Geometry: final body of the model. Coordinates: model frame, mm. Give positions to 0.01 mm unless a question says otherwise; leave off trailing zeros. Write each loop counter-clockwise with the first axis right and the second up, starting at its lowest first coordinate (ties: lowest second). Pieces come first, ordered by that corner, then holes.
Q1. Pin query (flat end, axial travel): pin 1 (1 mm diameter, centred on y = -37.5, z = 1, fed in from -X); pin 2 (0.6 mm diameter, centred on y = -33.5, z = 0.5, fed in from +X); pin 3 (0.6 mm diameter, centred on x = 16, z = 1.5, fed in from -Y). Return the tip coordinate at first contact, or that it passes through.
Q2. Line query: L1, parallel to Y at x = -22, z = 1.4; L2, parallel to X at y = -3.5, z = 0.5; L3, parallel to Y at x = 15, z = 0.5. Output: solid intervals per line, ascending.
Q3. Cut plane A-A on x = -16.5. Return the cut outline in (y, z).
Q4. Cut plane B-B on x = -22. Return the cut outline in (y, z).
Q5. Cut plane C-C on y = 2. Return the cut outline in (x, z).
Q6. Cut plane D-D on z = 1.35. Count the separate pieces of the cut face and the enclosed holes in it, plus the area to 3 significant figures.
```python
from build123d import *

# Parameters (mm, degrees)
F0_R     = 0.6
F0_R_2   = 0.85
F1_DEPTH = 2
F2_R     = 1


# Not quite as in the source:
# - a feature names something its author has since deleted; it is built from what else it names


with BuildPart() as f1:
    # F0 (on Top) → F1 (new body)
    with BuildSketch(Plane.XY):
        with BuildLine():
            ThreePointArc((-5.75, -27.5638593384), (-6.75, -27.25), (-7.75, -27.5638593384))
            Line((-7.75, -27.5638593384), (-7.75, -30.4361406616))
            ThreePointArc((-7.75, -30.4361406616), (-6.75, -30.75), (-5.75, -30.4361406616))
            Line((-5.75, -30.4361406616), (-5.75, -27.5638593384))
        make_face()
        with Locations((-6.75, -29)):
            Circle(F0_R, mode=Mode.SUBTRACT)
        with BuildLine():
            Line((-7.75, -30.4361406616), (-7.75, -27.5638593384))
            ThreePointArc((-7.75, -27.5638593384), (-8.5, -29), (-7.75, -30.4361406616))
        make_face()
        with BuildLine():
            ThreePointArc((-5.75, -30.4361406616), (-6.75, -30.75), (-7.75, -30.4361406616))
            Line((-7.75, -30.4361406616), (-7.75, -39.5638593384))
            ThreePointArc((-7.75, -39.5638593384), (-6.75, -39.25), (-5.75, -39.5638593384))
            Line((-5.75, -39.5638593384), (-5.75, -30.4361406616))
        make_face()
        with BuildLine():
            Line((-7.75, -42.4361406616), (-7.75, -39.5638593384))
            ThreePointArc((-7.75, -39.5638593384), (-8.5, -41), (-7.75, -42.4361406616))
        make_face()
        with BuildLine():
            ThreePointArc((-5.75, -39.5638593384), (-6.75, -39.25), (-7.75, -39.5638593384))
            Line((-7.75, -39.5638593384), (-7.75, -42.4361406616))
            ThreePointArc((-7.75, -42.4361406616), (-6.75, -42.75), (-5.75, -42.4361406616))
            Line((-5.75, -42.4361406616), (-5.75, -39.5638593384))
        make_face()
        with Locations((-6.75, -41)):
            Circle(F0_R, mode=Mode.SUBTRACT)
        with BuildLine():
            ThreePointArc((-5.75, -42.4361406616), (-6.75, -42.75), (-7.75, -42.4361406616))
            Line((-7.75, -42.4361406616), (-7.75, -46.5))
            Line((-7.75, -46.5), (7.75, -46.5))
            Line((7.75, -46.5), (7.75, -42.4361406616))
            ThreePointArc((7.75, -42.4361406616), (6.75, -42.75), (5.75, -42.4361406616))
            Line((5.75, -42.4361406616), (5.75, -45))
            Line((5.75, -45), (-5.75, -45))
            Line((-5.75, -45), (-5.75, -42.4361406616))
        make_face()
        with BuildLine():
            Line((7.75, -30.4361406616), (7.75, -27.5638593384))
            ThreePointArc((7.75, -27.5638593384), (6.75, -27.25), (5.75, -27.5638593384))
            Line((5.75, -27.5638593384), (5.75, -30.4361406616))
            ThreePointArc((5.75, -30.4361406616), (6.75, -30.75), (7.75, -30.4361406616))
        make_face()
        with Locations((6.75, -29)):
            Circle(F0_R, mode=Mode.SUBTRACT)
        with BuildLine():
            ThreePointArc((8.5, -29), (8.3012092057, -28.1899074127), (7.75, -27.5638593384))
            Line((7.75, -27.5638593384), (7.75, -30.4361406616))
            ThreePointArc((7.75, -30.4361406616), (8.3012092057, -29.8100925873), (8.5, -29))
        make_face()
        with BuildLine():
            Line((7.75, -39.5638593384), (7.75, -30.4361406616))
            ThreePointArc((7.75, -30.4361406616), (6.75, -30.75), (5.75, -30.4361406616))
            Line((5.75, -30.4361406616), (5.75, -39.5638593384))
            ThreePointArc((5.75, -39.5638593384), (6.75, -39.25), (7.75, -39.5638593384))
        make_face()
        with BuildLine():
            Line((7.75, -42.4361406616), (7.75, -39.5638593384))
            ThreePointArc((7.75, -39.5638593384), (6.75, -39.25), (5.75, -39.5638593384))
            Line((5.75, -39.5638593384), (5.75, -42.4361406616))
            ThreePointArc((5.75, -42.4361406616), (6.75, -42.75), (7.75, -42.4361406616))
        make_face()
        with Locations((6.75, -41)):
            Circle(F0_R, mode=Mode.SUBTRACT)
        with BuildLine():
            ThreePointArc((8.5, -41), (8.3012092057, -40.1899074127), (7.75, -39.5638593384))
            Line((7.75, -39.5638593384), (7.75, -42.4361406616))
            ThreePointArc((7.75, -42.4361406616), (8.3012092057, -41.8100925873), (8.5, -41))
        make_face()
        with BuildLine():
            ThreePointArc((-20, -8), (-20.0681483474, -8.5176380902), (-20.2679491924, -9))
            Line((-20.2679491924, -9), (-7.75, -9))
            Line((-7.75, -9), (-5.75, -9))
            Line((-5.75, -9), (5.75, -9))
            Line((5.75, -9), (7.75, -9))
            Line((7.75, -9), (20.2679491924, -9))
            ThreePointArc((20.2679491924, -9), (20, -8), (20.2679491924, -7))
            Line((20.2679491924, -7), (-20.2679491924, -7))
            ThreePointArc((-20.2679491924, -7), (-20.0681483474, -7.4823619098), (-20, -8))
        make_face()
        with BuildLine():
            ThreePointArc((24, -8), (23.7320508076, -7), (23, -6.2679491924))
            Line((23, -6.2679491924), (23, -9))
            Line((23, -9), (20.2679491924, -9))
            ThreePointArc((20.2679491924, -9), (22.5176380902, -9.9318516526), (24, -8))
        make_face()
        with BuildLine():
            ThreePointArc((23, -6.2679491924), (22, -6), (21, -6.2679491924))
            Line((21, -6.2679491924), (21, -7))
            Line((21, -7), (20.2679491924, -7))
            ThreePointArc((20.2679491924, -7), (20, -8), (20.2679491924, -9))
            Line((20.2679491924, -9), (23, -9))
            Line((23, -9), (23, -6.2679491924))
        make_face()
        with Locations((22, -8)):
            Circle(F0_R_2, mode=Mode.SUBTRACT)
        with BuildLine():
            ThreePointArc((23, 6.2679491924), (22, 6), (21, 6.2679491924))
            Line((21, 6.2679491924), (21, -6.2679491924))
            ThreePointArc((21, -6.2679491924), (22, -6), (23, -6.2679491924))
            Line((23, -6.2679491924), (23, 6.2679491924))
        make_face()
        with BuildLine():
            Line((21, -7), (21, -6.2679491924))
            ThreePointArc((21, -6.2679491924), (20.5857864376, -6.5857864376), (20.2679491924, -7))
            Line((20.2679491924, -7), (21, -7))
        make_face()
        with BuildLine():
            Line((21, 7), (20.2679491924, 7))
            ThreePointArc((20.2679491924, 7), (20.5857864376, 6.5857864376), (21, 6.2679491924))
            Line((21, 6.2679491924), (21, 7))
        make_face()
        with BuildLine():
            Line((23, 9), (20.2679491924, 9))
            ThreePointArc((20.2679491924, 9), (20, 8), (20.2679491924, 7))
            Line((20.2679491924, 7), (21, 7))
            Line((21, 7), (21, 6.2679491924))
            ThreePointArc((21, 6.2679491924), (22, 6), (23, 6.2679491924))
            Line((23, 6.2679491924), (23, 9))
        make_face()
        with Locations((22, 8)):
            Circle(F0_R_2, mode=Mode.SUBTRACT)
        with BuildLine():
            ThreePointArc((24, 8), (22.5176380902, 9.9318516526), (20.2679491924, 9))
            Line((20.2679491924, 9), (23, 9))
            Line((23, 9), (23, 6.2679491924))
            ThreePointArc((23, 6.2679491924), (23.7320508076, 7), (24, 8))
        make_face()
        with BuildLine():
            ThreePointArc((-20.2679491924, 9), (-20.0681483474, 8.5176380902), (-20, 8))
            ThreePointArc((-20, 8), (-20.0681483474, 7.4823619098), (-20.2679491924, 7))
            Line((-20.2679491924, 7), (20.2679491924, 7))
            ThreePointArc((20.2679491924, 7), (20, 8), (20.2679491924, 9))
            Line((20.2679491924, 9), (-20.2679491924, 9))
        make_face()
        with BuildLine():
            ThreePointArc((-21, -6.2679491924), (-22, -6), (-23, -6.2679491924))
            Line((-23, -6.2679491924), (-23, -9))
            Line((-23, -9), (-20.2679491924, -9))
            ThreePointArc((-20.2679491924, -9), (-20.0681483474, -8.5176380902), (-20, -8))
            ThreePointArc((-20, -8), (-20.0681483474, -7.4823619098), (-20.2679491924, -7))
            Line((-20.2679491924, -7), (-21, -7))
            Line((-21, -7), (-21, -6.2679491924))
        make_face()
        with Locations((-22, -8)):
            Circle(F0_R_2, mode=Mode.SUBTRACT)
        with BuildLine():
            Line((-23, -9), (-23, -6.2679491924))
            ThreePointArc((-23, -6.2679491924), (-23.4142135624, -9.4142135624), (-20.2679491924, -9))
            Line((-20.2679491924, -9), (-23, -9))
        make_face()
        with BuildLine():
            ThreePointArc((-20.2679491924, -7), (-20.5857864376, -6.5857864376), (-21, -6.2679491924))
            Line((-21, -6.2679491924), (-21, -7))
            Line((-21, -7), (-20.2679491924, -7))
        make_face()
        with BuildLine():
            Line((-23, 9), (-20.2679491924, 9))
            ThreePointArc((-20.2679491924, 9), (-23.4142135624, 9.4142135624), (-23, 6.2679491924))
            Line((-23, 6.2679491924), (-23, 9))
        make_face()
        with BuildLine():
            ThreePointArc((-20.2679491924, 7), (-20.0681483474, 7.4823619098), (-20, 8))
            ThreePointArc((-20, 8), (-20.0681483474, 8.5176380902), (-20.2679491924, 9))
            Line((-20.2679491924, 9), (-23, 9))
            Line((-23, 9), (-23, 6.2679491924))
            ThreePointArc((-23, 6.2679491924), (-22, 6), (-21, 6.2679491924))
            Line((-21, 6.2679491924), (-21, 7))
            Line((-21, 7), (-20.2679491924, 7))
        make_face()
        with Locations((-22, 8)):
            Circle(F0_R_2, mode=Mode.SUBTRACT)
        with BuildLine():
            ThreePointArc((-21, 6.2679491924), (-20.5857864376, 6.5857864376), (-20.2679491924, 7))
            Line((-20.2679491924, 7), (-21, 7))
            Line((-21, 7), (-21, 6.2679491924))
        make_face()
        with BuildLine():
            ThreePointArc((-21, 6.2679491924), (-22, 6), (-23, 6.2679491924))
            Line((-23, 6.2679491924), (-23, -6.2679491924))
            ThreePointArc((-23, -6.2679491924), (-22, -6), (-21, -6.2679491924))
            Line((-21, -6.2679491924), (-21, 6.2679491924))
        make_face()
        with BuildLine():
            Line((7.75, -9), (5.75, -9))
            Line((5.75, -9), (5.75, -14.3142581873))
            Line((5.75, -14.3142581873), (5.75, -15.422623174))
            Line((5.75, -15.422623174), (5.75, -20.073895466))
            Line((5.75, -20.073895466), (5.75, -21.1929723705))
            Line((5.75, -21.1929723705), (5.75, -27.5638593384))
            ThreePointArc((5.75, -27.5638593384), (6.75, -27.25), (7.75, -27.5638593384))
            Line((7.75, -27.5638593384), (7.75, -9))
        make_face()
        Polygon((5.75, -20.073895466), (1.0053343494, -17.6905184824), (-0.1362126115, -18.2361647275), (5.75, -21.1929723705), align=None)
        Polygon((5.75, -15.422623174), (5.75, -14.3142581873), (-0.125285608, -17.1225767595), (1.0053343494, -17.6905184824), align=None)
        Polygon((1.0053343494, -17.6905184824), (-0.125285608, -17.1225767595), (-1.2668325689, -17.6682230047), (-0.1362126115, -18.2361647275), align=None)
        Polygon((-5.75, -19.8111251883), (-5.75, -20.9194901751), (-0.1362126115, -18.2361647275), (-1.2668325689, -17.6682230047), align=None)
        Polygon((-0.125285608, -17.1225767595), (-5.75, -14.2971269157), (-5.75, -15.4162038202), (-1.2668325689, -17.6682230047), align=None)
        with BuildLine():
            Line((-5.75, -9), (-7.75, -9))
            Line((-7.75, -9), (-7.75, -27.5638593384))
            ThreePointArc((-7.75, -27.5638593384), (-6.75, -27.25), (-5.75, -27.5638593384))
            Line((-5.75, -27.5638593384), (-5.75, -20.9194901751))
            Line((-5.75, -20.9194901751), (-5.75, -19.8111251883))
            Line((-5.75, -19.8111251883), (-5.75, -15.4162038202))
            Line((-5.75, -15.4162038202), (-5.75, -14.2971269157))
            Line((-5.75, -14.2971269157), (-5.75, -9))
        make_face()
    extrude(amount=F1_DEPTH)

    # F2
    f2_edges = [f1.edges().sort_by_distance(p)[0] for p in [
        (-7.75, -46.5, 1),
        (7.75, -46.5, 1),
        (-5.75, -45, 1),
        (5.75, -45, 1),
        (-5.75, -20.91949, 1),
        (5.75, -21.192972, 1),
        (5.75, -20.073895, 1),
        (5.75, -15.422623, 1),
        (1.005334, -17.690518, 1),
        (-1.266833, -17.668223, 1),
        (-5.75, -14.297127, 1),
        (5.75, -14.314258, 1),
        (5.75, -9, 1),
        (-5.75, -9, 1),
        (-7.75, -9, 1),
        (7.75, -9, 1),
    ]]
    fillet(f2_edges, radius=F2_R)


solid = f1.part
```
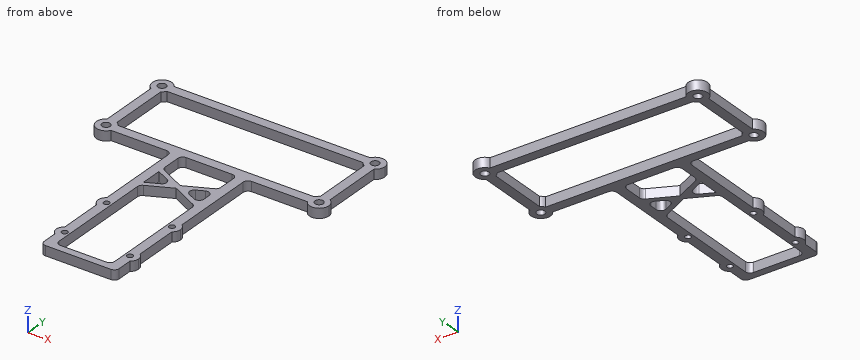
Data:
1. pin 1: stops at x = -7.75
1. pin 2: stops at x = 7.75
1. pin 3: stops at y = -9
2. L1: y = -10 to -8.85, -7.15 to 7.15, 8.85 to 10
2. L2: x = -23 to -21, 21 to 23
2. L3: y = -9 to -7, 7 to 9
3. outline: (-9, 0) - (-7, 0) - (-7, 2) - (-9, 2) - close; (7, 0) - (9, 0) - (9, 2) - (7, 2) - close
4. outline: (-10, 0) - (-8.85, 0) - (-8.85, 2) - (-10, 2) - close; (-7.15, 0) - (7.15, 0) - (7.15, 2) - (-7.15, 2) - close; (8.85, 0) - (10, 0) - (10, 2) - (8.85, 2) - close
5. outline: (-23, 0) - (-21, 0) - (-21, 2) - (-23, 2) - close; (21, 0) - (23, 0) - (23, 2) - (21, 2) - close
6. separate pieces: 1
6. enclosed holes: 13
6. area: 448 mm2
